Check sheet for the modelled part. Datum: model origin and axes. Units: mm. A direction names the side the tool comes from. Coordinates: 2 decimals unless noted, no trailing zeros. Write each loop counter-clockwise with the first axis right and the second up, starting at its lowest first coordinate (ties: lowest second). Pieces come first, ordered by that corner, then holes. Notation, with made-up numbers: (-28.5, 58.25) - (-10.5, 58.25) arc R27 ccw to (-10.5, 96.25) - close; hole circle Ø5 at (-8.75, 87.25). An arc over 180 degrees is marked (long way). Write each question's results on one line, items separated by ' | '.
from build123d import *

# Parameters (mm, degrees)
SKETCH_W        = 6.1
SKETCH_H        = 25
PAD_DEPTH       = 10
SKETCH001_R     = 1
PAD001_DEPTH    = 2
CHAMFER_SIZE    = 0.2
PAD002_DEPTH    = 10
SKETCH003_W     = 2
SKETCH003_H     = 20
SKETCH003_W_2   = 24.5
SKETCH003_H_2   = 2
PAD003_DEPTH    = 10
CHAMFER001_SIZE = 1.5


with BuildPart() as part:
    # Sketch → Pad (new body)
    with BuildSketch(Plane.XY):
        with Locations((3.05, 12.5)):
            Rectangle(SKETCH_W, SKETCH_H)
    extrude(amount=PAD_DEPTH)

    # Sketch001 (on Face6 of Pad) → Pad001 (join)
    with BuildSketch(Plane.XY.offset(10)):
        with Locations((1.7, 23.3)):
            Circle(SKETCH001_R)
        with Locations((1.7, 20.6)):
            Circle(SKETCH001_R)
        with Locations((1.7, 17.9)):
            Circle(SKETCH001_R)
        with Locations((1.7, 15.2)):
            Circle(SKETCH001_R)
        with Locations((1.7, 12.5)):
            Circle(SKETCH001_R)
        with Locations((1.7, 9.8)):
            Circle(SKETCH001_R)
        with Locations((1.7, 7.1)):
            Circle(SKETCH001_R)
        with Locations((1.7, 4.4)):
            Circle(SKETCH001_R)
        with Locations((1.7, 1.7)):
            Circle(SKETCH001_R)
        with Locations((4.4, 23.3)):
            Circle(SKETCH001_R)
        with Locations((4.4, 20.6)):
            Circle(SKETCH001_R)
        with Locations((4.4, 17.9)):
            Circle(SKETCH001_R)
        with Locations((4.4, 15.2)):
            Circle(SKETCH001_R)
        with Locations((4.4, 12.5)):
            Circle(SKETCH001_R)
        with Locations((4.4, 9.8)):
            Circle(SKETCH001_R)
        with Locations((4.4, 7.1)):
            Circle(SKETCH001_R)
        with Locations((4.4, 4.4)):
            Circle(SKETCH001_R)
        with Locations((4.4, 1.7)):
            Circle(SKETCH001_R)
    extrude(amount=PAD001_DEPTH)

    # Chamfer
    chamfer_edges = [part.edges().sort_by_distance(p)[0] for p in [
        (0.7, 15.2, 12),
        (3.4, 15.2, 12),
        (3.4, 12.5, 12),
        (0.7, 12.5, 12),
        (0.7, 9.8, 12),
        (3.4, 9.8, 12),
        (3.4, 7.1, 12),
        (0.7, 7.1, 12),
        (0.7, 4.4, 12),
        (3.4, 4.4, 12),
        (3.4, 1.7, 12),
        (0.7, 1.7, 12),
        (0.7, 17.9, 12),
        (3.4, 17.9, 12),
        (3.4, 20.6, 12),
        (0.7, 20.6, 12),
        (0.7, 23.3, 12),
        (3.4, 23.3, 12),
    ]]
    chamfer(chamfer_edges, length=CHAMFER_SIZE)

    # Sketch002 (on Face3 of Chamfer) → Pad002 (join)
    with BuildSketch(Plane.XY.offset(10)):
        Polygon((0, 25), (0, 0), (-8.581457, 0), (-8.581457, 31), (15.918543, 31), (15.918543, 0), (6.1, 0), (6.1, 25), align=None)
    extrude(amount=-PAD002_DEPTH)

    # Sketch003 (on Face5 of Pad002) → Pad003 (join)
    with BuildSketch(Plane.XY.offset(10)):
        with Locations((-7.597696, 10)):
            Rectangle(SKETCH003_W, SKETCH003_H)
        with Locations((3.67, 30)):
            Rectangle(SKETCH003_W_2, SKETCH003_H_2)
        with Locations((14.902304, 10)):
            Rectangle(SKETCH003_W, SKETCH003_H)
    extrude(amount=PAD003_DEPTH)

    # Chamfer001
    chamfer001_edges = [part.edges().sort_by_distance(p)[0] for p in [
        (13.902304, 10, 20),
        (-6.597696, 10, 20),
        (3.67, 29, 20),
    ]]
    chamfer(chamfer001_edges, length=CHAMFER001_SIZE)


solid = part.part
1. Sectioned sample at B-B (y = 20.6). Record the cut outline in (x, z).
Values follow:
outline: (-8.58, 0) - (15.92, 0) - (15.92, 10) - (5.4, 10) - (5.4, 11.8) - (5.2, 12) - (3.6, 12) - (3.4, 11.8) - (3.4, 10) - (2.7, 10) - (2.7, 11.8) - (2.5, 12) - (0.9, 12) - (0.7, 11.8) - (0.7, 10) - (-8.58, 10) - close
2. Access from +Z, -Z, +X, -X, +Y, -Y to the whole of each face (thin tool, end or side, straight path). Record for faces 1 (the flat face through (3, 29, 14)), 2 (the flat face through (15, 20, 15)), 3 (the flat face through (2, 7, 12)).
Values follow:
face 1: +Z, +X, -X | face 2: +Z, +X | face 3: +Z, -Y
3. Go/stop test with flat-tipped pins: pin 1 (0.5 mm diameter, centred on x = 4.5, y = 23.5, fed in from +Z); pin 2 (4 mm diameter, centred on y = 7, z = 12.5, fed in from +X); pin 3 (4 mm diameter, centred on x = -2.5, y = 23, fed in from +Z). Record where each tip stops, or that it passes through.
Values follow:
pin 1: stops at z = 12 | pin 2: stops at x = 15.9 | pin 3: stops at z = 10
4. Sectioned sample at A-A (z = 14). Record the cut outline in (x, y), then the cut area to 3 significant figures.
Values follow:
outline: (-8.6, 0) - (-6.6, 0) - (-6.6, 20) - (-8.6, 20) - close; (-8.58, 29) - (15.92, 29) - (15.92, 31) - (-8.58, 31) - close; (13.9, 0) - (15.9, 0) - (15.9, 20) - (13.9, 20) - close | area: 129 mm^2
5. Draft check along X on faces 4 (the flat face through (4, 23, 12)), 5 (the flat face through (4, 7, 12)), 6 (the flat face through (15.92, 30, 15)), 7 (the cylindrical face through (4.86, 3.51, 10.89)). Enter one of: pulls with the +X half, pulls with the -X half, needs draft (parallel to the pull), parting line crosses it, or undercut.
Values follow:
face 4: needs draft | face 5: undercut | face 6: pulls with the +X half | face 7: undercut
6. Sectioned sample at C-C (x = 6.5). Record the cut outline in (y, z).
Values follow:
outline: (0, 0) - (31, 0) - (31, 20) - (30.5, 20) - (29, 18.5) - (29, 10) - (0, 10) - close
7. Material ranges on L1, parallel to X at y = 7, z = 13.5; L2, parallel to Y at x = -7, z = 10.5; L3, parallel to Y at x = -4.5, z = 16.5, recorded low to high. Write a range as [from, to].
Values follow:
L1: x = [-8.6, -6.6], [13.9, 15.9] | L2: y = [0, 20], [29, 31] | L3: y = [29, 31]
